from build123d import *

# Parameters (mm, degrees)
SKETCH_1_W      = 10
SKETCH_1_H      = 3
SKETCH_1_W_2    = 3
SKETCH_1_H_2    = 10
EXTRUDE_1_DEPTH = 3


with BuildPart() as part:
    # 草图1 → 凸台-拉伸1 (new body)
    with BuildSketch(Plane.XY):
        Polygon((-22.5, 15), (-15.5, 15), (-15.5, 18), (-5.5, 18), (-5.5, 15), (5.5, 15), (5.5, 18), (15.5, 18), (15.5, 15), (22.5, 15), (22.5, -15), (22.5, -20), (-22.5, -20), (-22.5, -15), align=None)
        with Locations((-10.5, -16.5)):
            Rectangle(SKETCH_1_W, SKETCH_1_H, mode=Mode.SUBTRACT)
        with Locations((-19, -7.5)):
            Rectangle(SKETCH_1_W_2, SKETCH_1_H_2, mode=Mode.SUBTRACT)
        with Locations((10.5, -16.5)):
            Rectangle(SKETCH_1_W, SKETCH_1_H, mode=Mode.SUBTRACT)
        with Locations((-19, 7.5)):
            Rectangle(SKETCH_1_W_2, SKETCH_1_H_2, mode=Mode.SUBTRACT)
        with Locations((19, -7.5)):
            Rectangle(SKETCH_1_W_2, SKETCH_1_H_2, mode=Mode.SUBTRACT)
        with Locations((19, 7.5)):
            Rectangle(SKETCH_1_W_2, SKETCH_1_H_2, mode=Mode.SUBTRACT)
    extrude(amount=EXTRUDE_1_DEPTH)


solid = part.part
Can you work these out from the model? Positions are in its coordinate system, mm. A direction names the side the tool comes from. Give positions to 0.01 mm unless a question says otherwise; leave off trailing zeros. Loops run counter-clockwise (first coordinate to the right, second up) from the corner with the lowest first, then second, coordinate; pieces in that order, holes last. Notation, with made-up numbers: (33.5, 86.5) - (89.5, 86.5) arc R18 ccw to (89.5, 116.5) - close; hole circle Ø7 at (57, 58.25). An arc over 180 degrees is marked (long way). One line per item, written item: value.
(1) If we section it at D-D, the plane x = 18: List the corners of the cut face in (y, z) for me, plus the area to 3 significant figures.
Verdict:
outline: (-20, 0) - (-12.5, 0) - (-12.5, 3) - (-20, 3) - close; (-2.5, 0) - (2.5, 0) - (2.5, 3) - (-2.5, 3) - close; (12.5, 0) - (15, 0) - (15, 3) - (12.5, 3) - close
area: 45.0 mm^2
(2) On a 3-axis mill with a long thin cutter (end or side, diameter ignored), from which of +Z, -Z, +X, -X, +Y, -Y can I reach the whole of each face in a straight line? I mean faces 1 (the face through (-5.5, 17, 1)), 2 (the face through (19, 12.5, 1)), 3 (the face through (15.5, 17, 1)), 4 (the face through (-15.5, 16, 1)). Say none if no direction works.
Verdict:
face 1: +Z, -Z, +Y
face 2: +Z, -Z
face 3: +Z, -Z, +X, +Y
face 4: +Z, -Z, -X, +Y
(3) If we section it at A-A, the plane y = 15.5: List the corners of the cut face in (x, z) for me.
Verdict:
outline: (-15.5, 0) - (-5.5, 0) - (-5.5, 3) - (-15.5, 3) - close; (5.5, 0) - (15.5, 0) - (15.5, 3) - (5.5, 3) - close
(4) I need wall thicknesses on line 1 along X through (y, z) = (-8.5, 0.65); line 2 along Y through (x, z) = (-7.5, 2.2); line 3 along Y through (x, z) = (19, 0.6). Which ranges of each line are inside material? Lowest first, please.
Verdict:
line 1: -22.5 to -20.5, -17.5 to 17.5, 20.5 to 22.5
line 2: -20 to -18, -15 to 18
line 3: -20 to -12.5, -2.5 to 2.5, 12.5 to 15
(5) I'm going to push flat-ended pins straight in: pin 1 (1 mm diameter, centred on x = 1.5, y = 7, fed in from -Z); pin 2 (0.9 mm diameter, centred on x = 2, z = 1, fed in from +Y); pin 3 (1.5 mm diameter, centred on y = 17, z = 1.5, fed in from +X). Where does each tip first touch, or does it pass through?
Verdict:
pin 1: z = 0
pin 2: y = 15
pin 3: x = 15.5
(6) If we section it at C-C, the plane y = -5: List the corners of the cut face in (x, z) for me, plus the area to 3 significant figures.
Verdict:
outline: (-22.5, 0) - (-20.5, 0) - (-20.5, 3) - (-22.5, 3) - close; (-17.5, 0) - (17.5, 0) - (17.5, 3) - (-17.5, 3) - close; (20.5, 0) - (22.5, 0) - (22.5, 3) - (20.5, 3) - close
area: 117 mm^2
(7) If we section it at B-B, the plane x = -15: List the corners of the cut face in (y, z) for me, plus the area to 3 significant figures.
Verdict:
outline: (-20, 0) - (-18, 0) - (-18, 3) - (-20, 3) - close; (-15, 0) - (18, 0) - (18, 3) - (-15, 3) - close
area: 105 mm^2
